from build123d import *

# Parameters (mm, degrees)
EXTRUDE_1_DEPTH             = 140
CUT_EXTRUDE_1_REACH         = 641.766
SKETCH_2_R                  = 190.25
SKETCH_3_R                  = 14
CUT_EXTRUDE_2_DEPTH         = 35
PATTERN_CIRCULAR_1_COUNT    = 8
MIRROR_1_COPY_1_SKETCH_R    = 14
MIRROR_1_COPY_1_DEPTH       = 35
MIRROR_1_COPY_2_SKETCH_R    = 14
MIRROR_1_COPY_2_DEPTH       = 35
MIRROR_1_COPY_3_SKETCH_R    = 14
MIRROR_1_COPY_3_DEPTH       = 35
MIRROR_1_COPY_4_SKETCH_R    = 14
MIRROR_1_COPY_4_DEPTH       = 35
MIRROR_1_COPY_5_SKETCH_R    = 14
MIRROR_1_COPY_5_DEPTH       = 35
MIRROR_1_COPY_6_SKETCH_R    = 14
MIRROR_1_COPY_6_DEPTH       = 35
MIRROR_1_COPY_7_SKETCH_R    = 14
MIRROR_1_COPY_7_DEPTH       = 35
SKETCH_4_R                  = 4.25
CUT_EXTRUDE_3_DEPTH         = 15
CUT_EXTRUDE_4_REACH         = 656.766
CUT_EXTRUDE_4_END_RADIUS    = 190.25
CUT_EXTRUDE_START           = -15
SKETCH_6_R                  = 4.5
CUT_EXTRUDE_5_REACH         = 587.491
SKETCH_7_R                  = 16
SKETCH_8_R                  = 24
CUT_EXTRUDE_6_DEPTH         = 30
PATTERN_LINEAR_1_COUNT      = 2
PATTERN_LINEAR_1_PITCH      = 600
PATTERN_LINEAR_1_COUNT_DIR2 = 2
PATTERN_LINEAR_1_PITCH_DIR2 = 75
CUT_EXTRUDE_7_REACH         = 587.491
SKETCH_7_3_R                = 10
PATTERN_LINEAR_2_COUNT      = 2
PATTERN_LINEAR_2_PITCH      = 660
FILLET_1_R                  = 25


with BuildPart() as part:
    # 草图1 → 凸台-拉伸1 (new body)
    with BuildSketch(Plane(origin=(0, 0, 0), x_dir=(1, 0, 0), z_dir=(0, 1, 0))):
        Polygon((360, 0), (-360, 0), (-360, 70), (-250, 70), (-250, 365), (-105, 510), (105, 510), (250, 365), (250, 70), (360, 70), align=None)
    extrude(amount=EXTRUDE_1_DEPTH)

    # 草图2 → 切除-拉伸1 (cut, up to next)
    with BuildSketch(Plane(origin=(0, 140, 0), x_dir=(1, 0, 0), z_dir=(0, 1, 0)), mode=Mode.PRIVATE) as cut_extrude_1_sk1:
        with Locations(Location((0, 260, 0), (0, 0, 270))):
            Circle(SKETCH_2_R)
    cut_extrude_1_tool1 = extrude(cut_extrude_1_sk1.sketch, amount=-CUT_EXTRUDE_1_REACH, mode=Mode.PRIVATE) & part.part
    add(cut_extrude_1_tool1.solids().sort_by_distance((0, 140, -260))[0], mode=Mode.SUBTRACT)

    # 草图3 → 切除-拉伸2 (cut)
    with BuildSketch(Plane(origin=(0, 140, 0), x_dir=(1, 0, 0), z_dir=(0, 1, 0))):
        with Locations(Location((-86.103772282, 467.872894815, 0), (0, 0, 270))):
            Circle(SKETCH_3_R)
    cut_extrude_2 = extrude(amount=-CUT_EXTRUDE_2_DEPTH, mode=Mode.SUBTRACT)

    # 阵列(圆周)1: 切除-拉伸2 ×8 about axis
    pattern_circular_1_axis = Axis((0, 0, -260), (0, 1, 0))
    for i in range(1, PATTERN_CIRCULAR_1_COUNT):
        add(cut_extrude_2.rotate(pattern_circular_1_axis, i * 360 / PATTERN_CIRCULAR_1_COUNT), mode=Mode.SUBTRACT)

    # 镜向1: 切除-拉伸2 across plane
    add(cut_extrude_2.mirror(Plane.ZX.offset(70)), mode=Mode.SUBTRACT)

    # 镜向1 copy 1 sketch → 镜向1 copy 1 (cut)
    with BuildSketch(Plane(origin=(183.847763109, 0, -76.152236891), x_dir=(0.7071067811865476, 0, -0.7071067811865475), z_dir=(0, -1, 0))):
        with Locations((-86.103772282, -467.872894815)):
            Circle(MIRROR_1_COPY_1_SKETCH_R)
    extrude(amount=-MIRROR_1_COPY_1_DEPTH, mode=Mode.SUBTRACT)

    # 镜向1 copy 2 sketch → 镜向1 copy 2 (cut)
    with BuildSketch(Plane(origin=(260, 0, -260), x_dir=(0, 0, -1), z_dir=(0, -1, 0))):
        with Locations((-86.103772282, -467.872894815)):
            Circle(MIRROR_1_COPY_2_SKETCH_R)
    extrude(amount=-MIRROR_1_COPY_2_DEPTH, mode=Mode.SUBTRACT)

    # 镜向1 copy 3 sketch → 镜向1 copy 3 (cut)
    with BuildSketch(Plane(origin=(183.847763109, 0, -443.847763109), x_dir=(-0.7071067811865475, 0, -0.7071067811865476), z_dir=(0, -1, 0))):
        with Locations((-86.103772282, -467.872894815)):
            Circle(MIRROR_1_COPY_3_SKETCH_R)
    extrude(amount=-MIRROR_1_COPY_3_DEPTH, mode=Mode.SUBTRACT)

    # 镜向1 copy 4 sketch → 镜向1 copy 4 (cut)
    with BuildSketch(Plane(origin=(0, 0, -520), x_dir=(-1, 0, 0), z_dir=(0, -1, 0))):
        with Locations((-86.103772282, -467.872894815)):
            Circle(MIRROR_1_COPY_4_SKETCH_R)
    extrude(amount=-MIRROR_1_COPY_4_DEPTH, mode=Mode.SUBTRACT)

    # 镜向1 copy 5 sketch → 镜向1 copy 5 (cut)
    with BuildSketch(Plane(origin=(-183.847763109, 0, -443.847763109), x_dir=(-0.7071067811865477, 0, 0.7071067811865475), z_dir=(0, -1, 0))):
        with Locations((-86.103772282, -467.872894815)):
            Circle(MIRROR_1_COPY_5_SKETCH_R)
    extrude(amount=-MIRROR_1_COPY_5_DEPTH, mode=Mode.SUBTRACT)

    # 镜向1 copy 6 sketch → 镜向1 copy 6 (cut)
    with BuildSketch(Plane(origin=(-260, 0, -260), x_dir=(0, 0, 1), z_dir=(0, -1, 0))):
        with Locations((-86.103772282, -467.872894815)):
            Circle(MIRROR_1_COPY_6_SKETCH_R)
    extrude(amount=-MIRROR_1_COPY_6_DEPTH, mode=Mode.SUBTRACT)

    # 镜向1 copy 7 sketch → 镜向1 copy 7 (cut)
    with BuildSketch(Plane(origin=(-183.847763109, 0, -76.152236891), x_dir=(0.7071067811865474, 0, 0.7071067811865477), z_dir=(0, -1, 0))):
        with Locations((-86.103772282, -467.872894815)):
            Circle(MIRROR_1_COPY_7_SKETCH_R)
    extrude(amount=-MIRROR_1_COPY_7_DEPTH, mode=Mode.SUBTRACT)

    # 草图4 → 切除-拉伸3 (cut)
    with BuildSketch(Plane(origin=(0, 0, -510), x_dir=(-1, 0, 0), z_dir=(0, 0, -1))):
        with Locations((0, 70)):
            Circle(SKETCH_4_R)
    extrude(amount=-CUT_EXTRUDE_3_DEPTH, mode=Mode.SUBTRACT)

    # 切除-拉伸4: up to this cylinder (the profile starts outside it)
    cut_extrude_4_end = Plane(origin=(0, 70, -260), z_dir=(0, 1, 0)) * Cylinder(CUT_EXTRUDE_4_END_RADIUS, 1695.032, mode=Mode.PRIVATE)
    # 草图6 → 切除-拉伸4 (cut, up to the surface)
    with BuildSketch(Plane(origin=(0, 0, -510), x_dir=(-1, 0, 0), z_dir=(0, 0, -1)).offset(CUT_EXTRUDE_START), mode=Mode.PRIVATE) as cut_extrude_4_sk1:
        with Locations((0, 70)):
            Circle(SKETCH_6_R)
    cut_extrude_4_tool1 = extrude(cut_extrude_4_sk1.sketch, amount=-CUT_EXTRUDE_4_REACH, mode=Mode.PRIVATE) - cut_extrude_4_end
    add(cut_extrude_4_tool1.solids().sort_by_distance((0, 70, -495))[0], mode=Mode.SUBTRACT)

    # 草图7 → 切除-拉伸5 (cut, up to next)
    with BuildSketch(Plane(origin=(0, 0, -70), x_dir=(-1, 0, 0), z_dir=(0, 0, -1)), mode=Mode.PRIVATE) as cut_extrude_5_sk1:
        with Locations((-300, 107.5)):
            Circle(SKETCH_7_R)
    cut_extrude_5_tool1 = extrude(cut_extrude_5_sk1.sketch, amount=-CUT_EXTRUDE_5_REACH, mode=Mode.PRIVATE) & part.part
    cut_extrude_5 = cut_extrude_5_tool1.solids().sort_by_distance((300, 107.5, -70))[0]
    add(cut_extrude_5, mode=Mode.SUBTRACT)

    # 草图8 → 切除-拉伸6 (cut)
    with BuildSketch(Plane(origin=(0, 0, -70), x_dir=(-1, 0, 0), z_dir=(0, 0, -1))):
        with Locations((-300, 107.5)):
            Circle(SKETCH_8_R)
    cut_extrude_6 = extrude(amount=-CUT_EXTRUDE_6_DEPTH, mode=Mode.SUBTRACT)

    # 阵列(线性)1: 切除-拉伸5, Cut-Extrude 6 2 × 2
    with Locations(*[(-i * PATTERN_LINEAR_1_PITCH, -j * PATTERN_LINEAR_1_PITCH_DIR2, 0) for i in range(PATTERN_LINEAR_1_COUNT) for j in range(PATTERN_LINEAR_1_COUNT_DIR2) if (i, j) != (0, 0)]):
        add(cut_extrude_5, mode=Mode.SUBTRACT)
        add(cut_extrude_6, mode=Mode.SUBTRACT)

    # 草图7<3> → 切除-拉伸7 (cut, up to next)
    with BuildSketch(Plane(origin=(0, 0, -70), x_dir=(-1, 0, 0), z_dir=(0, 0, -1)), mode=Mode.PRIVATE) as cut_extrude_7_sk1:
        with Locations((-330, 70)):
            Circle(SKETCH_7_3_R)
    cut_extrude_7_tool1 = extrude(cut_extrude_7_sk1.sketch, amount=-CUT_EXTRUDE_7_REACH, mode=Mode.PRIVATE) & part.part
    cut_extrude_7 = cut_extrude_7_tool1.solids().sort_by_distance((330, 70, -70))[0]
    add(cut_extrude_7, mode=Mode.SUBTRACT)

    # 阵列(线性)2: 切除-拉伸7 ×2
    with Locations(*[(-i * PATTERN_LINEAR_2_PITCH, 0, 0) for i in range(1, PATTERN_LINEAR_2_COUNT)]):
        add(cut_extrude_7, mode=Mode.SUBTRACT)

    # 圆角1
    fillet_1_edges = [part.edges().sort_by_distance(p)[0] for p in [
        (-250, 70, -70),
        (250, 70, -70),
    ]]
    fillet(fillet_1_edges, radius=FILLET_1_R)


solid = part.part
Work out the finished part from the listing and answer in its coordinate system (mm). A direction names the side the tool comes from. Coordinates: 2 decimals unless noted, no trailing zeros. Write each loop counter-clockwise with the first axis right and the second up, starting at its lowest first coordinate (ties: lowest second). Pieces come first, ordered by that corner, then holes. Notation, with made-up numbers: M 5,18.25 L 22,18.25 A6 cw 22,25.25 Z; hole C 74,51.25 d10. An arc over 180 degrees is marked long. Answer as CSV lines item,"result". Start each with the question number.
Item 1: Flat-ended cylindrical pins translate along their axes: P1, Ø23, axis at x = 330, y = 70, coming from the -Z side; P2, Ø14, axis at x = -90.5, z = -465, coming from the +Y side; P3, Ø25, axis at x = 86.1, z = -467.87, coming from the -Y side. Find the tip coordinate at first contact, or state that the pin passes through.
Item 2: Determine the mould class of faces 5 (the face through (-316, 103, -40)), 6 (the face through (-208, 35, -174)), 7 (the face through (360, 69, -35)) for opening direction Y: released by +Y, released by -Y, zero draft, split by the parting line, or undercut.
Item 3: Consider L1, parallel to Y at x = 300, z = -62.5; L2, parallel to X at y = 85.5, z = -257.5; L3, parallel to Z at x = -212, y = 115. Determine where each line is inside the solid, lowest interval first.
Item 4: A tool of negligible diameter and unlimited length cuts with its end or side. For faces 1 (the face through (208, 35, -346)), 2 (the face through (-76.64, 122.74, -478.19)), 3 (the face through (323.977, 33.555, -55.21)), 4 (the face through (317, 69, -70)), from which of +Z, -Z, +X, -X, +Y, -Y can it reach the whole face along a straight path? Write none if from no direction.
Item 5: Section A-A on x = 300 is taken. Write down the section's boundary in (y, z), and give its area (3 significant figures).
Item 6: Section B-B on x = -32 is taken. Write down the section's boundary in (y, z).
Item 7: Section C-C on z = -406 is taken. Write down the section's boundary in (x, y), and give its area (3 significant figures).
Checks:
1,P1,"stops at z = -70"
1,P2,"stops at y = 105"
1,P3,"stops at y = 35"
2,face 5,"undercut"
2,face 6,"released by -Y"
2,face 7,"zero draft"
3,L1,"y = 0 to 8.5, 56.5 to 83.5, 131.5 to 140"
3,L2,"x = -250 to -190.23, 190.23 to 250"
3,L3,"z = -403 to -359.48, -332.73 to -187.27, -160.52 to 0"
4,face 1,"-Y"
4,face 2,"+Y"
4,face 3,"-Z"
4,face 4,"-Z, +X, +Y, -Y"
5,outline,"M 0,-70 L 8.5,-70 L 8.5,-40 L 16.5,-40 L 16.5,0 L 0,0 Z; M 48.5,-40 L 56.5,-40 L 56.5,-70 L 83.5,-70 L 83.5,-40 L 91.5,-40 L 91.5,0 L 48.5,0 Z; M 123.5,-40 L 131.5,-40 L 131.5,-70 L 140,-70 L 140,0 L 123.5,0 Z"
5,area,"4,360 mm²"
6,outline,"M 0,-510 L 140,-510 L 140,-447.54 L 0,-447.54 Z; M 0,-72.46 L 140,-72.46 L 140,0 L 0,0 Z"
7,outline,"M -209,0 L -121.98,0 L -121.98,140 L -209,140 Z; M 121.98,0 L 209,0 L 209,140 L 121.98,140 Z"
7,area,"24,400 mm²"
